```python
from build123d import *

# Parameters (mm, degrees)
F0_W     = 482.6
F0_H     = 533.4
F1_DEPTH = 762
F2_R     = 25.4
F3_T     = -2.54


# Not quite as in the source:
# - a shell that OpenCascade refuses in one call is made with other operations: the cavity is built on its own and cut out


with BuildPart() as f1:
    # F0 (on Front) → F1 (new body)
    with BuildSketch(Plane.XZ):
        with Locations((241.3, 266.7)):
            Rectangle(F0_W, F0_H)
    extrude(amount=F1_DEPTH)

    # F2
    f2_edges = [f1.edges().sort_by_distance(p)[0] for p in [
        (482.6, -381, 533.4),
        (482.6, -762, 266.7),
        (0, -381, 533.4),
        (241.3, 0, 533.4),
        (241.3, -762, 533.4),
        (241.3, -762, 0),
        (482.6, -381, 0),
        (482.6, 0, 266.7),
        (0, 0, 266.7),
        (241.3, 0, 0),
        (0, -381, 0),
        (0, -762, 266.7),
    ]]
    fillet(f2_edges, radius=F2_R)

    # F3: a shell. OpenCascade refuses it in one call, so the cavity is built on its own and cut out:
    # the body offset inwards by the wall thickness, plus a prism from it out through each open face.
    f3_core = offset(f1.part, amount=F3_T, mode=Mode.PRIVATE)
    f3_exits = [f3_core.faces().sort_by_distance(p)[0] for p in [
        (241.3, -2.54, 266.7),
        (241.3, -759.46, 266.7),
        (480.06, -381, 266.7),
        (241.3, -381, 530.86),
        (2.54, -381, 266.7),
    ]]
    add(f3_core, mode=Mode.SUBTRACT)
    extrude(f3_exits, amount=-F3_T, mode=Mode.SUBTRACT)


solid = f1.part
```
Source: CAD feature listing. Evaluate the final solid. Frame: model axes, mm. A direction names the side the tool comes from. Coordinates: 2 decimals unless noted, no trailing zeros. Write each loop counter-clockwise with the first axis right and the second up, starting at its lowest first coordinate (ties: lowest second). Pieces come first, ordered by that corner, then holes. Notation, with made-up numbers: M 35,-10 L 61,-10 A18 ccw 61,-4 Z; hole C 2.25,10 d3. An arc over 180 degrees is marked long. Answer as a JSON object with one key per item and string values.
1. Draft query along X for faces 1 (the cylindrical face through (244.323, -752.586, 524.341)), 2 (the cylindrical face through (474.96, -385.98, 7.24)), 3 (the cylindrical face through (7.24, -7.64, 270.08)), 4 (the cylindrical face through (244.32, -7.64, 526.16)). Return one class per face: released by +X, released by -X, zero draft, split by the parting line, or undercut.
Evaluation:
{"face 1": "undercut", "face 2": "released by +X", "face 3": "released by -X", "face 4": "zero draft"}
2. Access query for faces 5 (the flat face through (238, -376, 2.54)), 6 (the cylindrical face through (9.059, -385.978, 9.414)), 7 (the cylindrical face through (244.32, -754.36, 526.16)). Directions: +Z, -Z, +X, -X, +Y, -Y. A direction counts if a zero-diameter tool reaches every point of the face in a straight line with its end or side. Return the directions, or none.
Evaluation:
{"face 5": "+Z", "face 6": "none", "face 7": "+Z, +X, -X, -Y"}
3. Cut plane B-B on y = -50.5. Output: boundary loops of the cut face in (x, z).
Evaluation:
{"outline": "M 0,25.4 A25.4 ccw 25.4,0 L 457.2,0 A25.4 ccw 482.6,25.4 L 480.06,25.4 A22.86 cw 457.2,2.54 L 25.4,2.54 A22.86 cw 2.54,25.4 Z; M 0,508 L 2.54,508 A22.86 cw 25.4,530.86 L 25.4,533.4 A25.4 ccw Z; M 457.2,530.86 A22.86 cw 480.06,508 L 482.6,508 A25.4 ccw 457.2,533.4 Z"}
4. Cut plane A-A on x = 209.5. Output: boundary loops of the cut face in (y, z), plus the area to 3 significant figures.
Evaluation:
{"outline": "M -762,25.4 A25.4 ccw -736.6,0 L -25.4,0 A25.4 ccw 0,25.4 L -2.54,25.4 A22.86 cw -25.4,2.54 L -736.6,2.54 A22.86 cw -759.46,25.4 Z; M -762,508 L -759.46,508 A22.86 cw -736.6,530.86 L -736.6,533.4 A25.4 ccw Z; M -25.4,530.86 A22.86 cw -2.54,508 L 0,508 A25.4 ccw -25.4,533.4 Z", "area": "2,190 mm^2"}
5. Contact query for flat-ended pins moving along their axis: P1, Ø2, axis at y = -386.5, z = 532, coming from the -X side; P2, Ø2, axis at x = 1, y = -371, coming from the +Z side; P3, Ø3, axis at x = 356, y = -129, coming from the +Z side. Output: stop coordinate, or through.
Evaluation:
{"P1": "x = 14.62", "P2": "z = 517.88", "P3": "z = 2.54"}
6. Ray query, L1, parallel to Z at x = 168, y = -250; L2, parallel to X at y = -262.5, z = 22; L3, parallel to Y at x = 462.5, z = 51. Return the intervals inside material, ascending.
Evaluation:
{"L1": "0 to 2.54", "L2": "0.23 to 2.79, 479.81 to 482.37", "L3": "-761.44 to -758.84, -3.16 to -0.56"}
7. Cut plane C-C on z = 142. Output: boundary loops of the cut face in (x, y), plus the area to 3 significant figures.
Evaluation:
{"outline": "M 0,-736.6 A25.4 ccw 25.4,-762 L 25.4,-759.46 A22.86 cw 2.54,-736.6 Z; M 0,-25.4 L 2.54,-25.4 A22.86 cw 25.4,-2.54 L 25.4,0 A25.4 ccw Z; M 457.2,-762 A25.4 ccw 482.6,-736.6 L 480.06,-736.6 A22.86 cw 457.2,-759.46 Z; M 457.2,-2.54 A22.86 cw 480.06,-25.4 L 482.6,-25.4 A25.4 ccw 457.2,0 Z", "area": "385 mm^2"}
